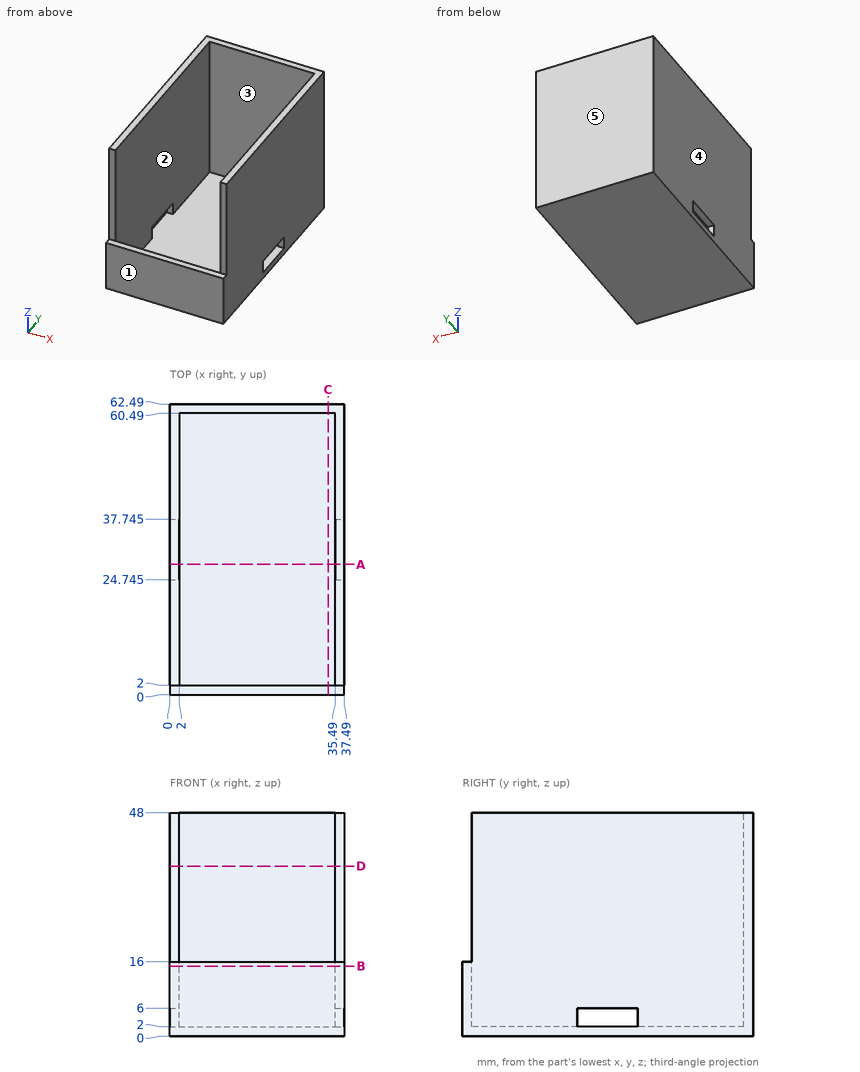
Design review of the part shown in the three views and the two pictorial views. Dimensions are in mm from the part's minimum x, y and z. A direction names the side the tool comes from. Round coordinates to 2 decimals unless told otherwise and drop trailing zeros. Loops run counter-clockwise (first coordinate to the right, second up) from the corner with the lowest first, then second, coordinate; pieces in that order, holes last. Notation, with made-up numbers: (-20.5, 35.25) -> (3.5, 35.25) arc R12 ccw to (3.5, 55.25) -> close; hole circle Ø8 at (-27, -5.5). An arc over 180 degrees is marked (long way). Use one line per item in the form item = value. Start each with the question number.
Q1. We need section A-A on y = 28. Give the boundary of the cut face in (x, z).
Q2. We need section B-B on z = 15. Give the boundary of the cut face in (x, y).
Q3. For pin 1 Ø11 at (x, y) = (10.5, 37) entering from +Z; pin 2 Ø1.6 at (x, z) = (0.5, 39.5) entering from -Y; pin 3 Ø8 at (x, z) = (23, 24.5) entering from -Y, all flat-tipped, find the tip position at first contact; note any pin that passes through.
Q4. Draft analysis for pull direction Y (two halves, no side actions). For the marked faces 3, 4 and 5, state which applies: +Y half, -Y half, draft (parallel to the pull), parting line (faces both ways), or undercut.
Q5. Wall thickness on line 1 along X through (y, z) = (51.5, 37); line 2 along Y through (x, z) = (19, 8); line 3 along Z through (x, y) = (36.5, 26.5): over which ranges is each line inside the solid? List them lowest first. Write a range as [from, to].
Q6. We need section D-D on z = 36.5. Give the boundary of the cut face in (x, y), then the cut area to 3 significant figures.
Q7. We need section C-C on x = 34. Give the boundary of the cut face in (y, z), then the cut area to 3 significant figures.
Q8. Machinability: for the marked faces 1 and 2, which of the approach directions +Z, -Z, +X, -X, +Y, -Y give a long, thin tool a straight path to every point of the face, cutting with its end or side? Answer none if there is none.
Calculated:
q1.outline = (0, 0) -> (37.49, 0) -> (37.49, 2) -> (0, 2) -> close; (0, 6) -> (2, 6) -> (2, 48) -> (0, 48) -> close; (35.49, 6) -> (37.49, 6) -> (37.49, 48) -> (35.49, 48) -> close
q2.outline = (0, 0) -> (37.49, 0) -> (37.49, 62.49) -> (0, 62.49) -> close; hole (2, 2) -> (35.49, 2) -> (35.49, 60.49) -> (2, 60.49) -> close
q3.pin_1 = 2
q3.pin_2 = 2
q3.pin_3 = 60.49
q4.face_3 = undercut
q4.face_4 = draft
q4.face_5 = +Y half
q5.line_1 = [0, 2], [35.49, 37.49]
q5.line_2 = [0, 2], [60.49, 62.49]
q5.line_3 = [0, 2], [6, 48]
q6.outline = (0, 2) -> (2, 2) -> (2, 60.49) -> (35.49, 60.49) -> (35.49, 2) -> (37.49, 2) -> (37.49, 62.49) -> (0, 62.49) -> close
q6.area = 309 mm²
q7.outline = (0, 0) -> (62.49, 0) -> (62.49, 48) -> (60.49, 48) -> (60.49, 2) -> (2, 2) -> (2, 16) -> (0, 16) -> close
q7.area = 245 mm²
q8.face_1 = +Z, -Z, +X, -X, -Y
q8.face_2 = +Z
